The listing builds one solid part. Answer for the finished solid, in the listing's coordinates (mm). A direction names the side the tool comes from. Round coordinates to 2 decimals unless told otherwise and drop trailing zeros. Write each loop counter-clockwise with the first axis right and the second up, starting at its lowest first coordinate (ties: lowest second). Pieces come first, ordered by that corner, then holes.
Item 1: Find section B-B on x = 15.5. Give the vertices of the cut face in (y, z).
Item 2: A tool of negligible diameter and unlimited length cuts with its end or side. For faces 5 (the face through (15.023, -37.648, 1.014)), 6 (the face through (0, 1, -1)), from which of +Z, -Z, +X, -X, +Y, -Y can it reach the whole face along a straight path? Write none if from no direction.
Item 3: Find section C-C on z = -0.45. Give the vertices of the cut face in (x, y), then the cut area to 3 significant figures.
Item 4: Each of these flat-tipped pins is pushed along its axis until it touches: pin 1 (0.8 mm diameter, centred on x = -5, z = -0.5, fed in from -Y); pin 2 (1.3 mm diameter, centred on x = -16.5, y = 35.5, fed in from +Z). Where does it stop, or does it pass through?
Item 5: Find section D-D on y = 9. Give the vertices of the cut face in (x, z), then the cut area to 3 significant figures.
Item 6: Find section A-A on y = -35.5. Give the vertices of the cut face in (x, z), then the cut area to 3 significant figures.
Item 7: Find the intervals of material crossed by probe 1 along X at (y, z) = (-13.5, -0.45); probe 2 along Z at (x, y) = (18, -25); probe 3 along Y at (x, z) = (-12, -0.15), in increasing order.
Item 8: For a pull along Y with two mould halves and no side action, classify faces 1 (the face through (-18, 0, 0)), 2 (the face through (0, 40, 1)), 3 (the face through (0, -40, 1)), 4 (the face through (-15.66, 36.69, -0.49)) as +Y half, -Y half, draft (parallel to the pull), parting line (faces both ways), or undercut.
```python
from build123d import *

# Parameters (mm, degrees)
ESQUISSE1_W             = 40
ESQUISSE1_H             = 80
ESQUISSE1_W_2           = 35.6
ESQUISSE1_H_2           = 75.6
BOSS_EXTRU_1_DEPTH      = 2
ESQUISSE1_3_W           = 35.6
ESQUISSE1_3_H           = 75.6
BOSS_EXTRU_2_DEPTH      = 1
ESQUISSE2_R             = 1.2
ENL_V_MAT_EXTRU_1_DEPTH = 45.821869662
ESQUISSE2_3_R           = 2.2
ESQUISSE2_3_R_2         = 1.2
ENL_V_MAT_EXTRU_2_DEPTH = 2


with BuildPart() as part:
    # Esquisse1 → Boss.-Extru.1 (new body)
    # profile 1 of 2: a face of its own
    with BuildSketch(Plane.XY):
        Rectangle(ESQUISSE1_W, ESQUISSE1_H)
        Rectangle(ESQUISSE1_W_2, ESQUISSE1_H_2, mode=Mode.SUBTRACT)
    # profile 2 of 2: a face of its own
    with BuildSketch(Plane.XY):
        Rectangle(ESQUISSE1_W_2, ESQUISSE1_H_2)
    extrude(amount=BOSS_EXTRU_1_DEPTH)

    # Esquisse1_3 → Boss.-Extru.2 (add)
    with BuildSketch(Plane.XY):
        Rectangle(ESQUISSE1_3_W, ESQUISSE1_3_H)
    extrude(amount=-BOSS_EXTRU_2_DEPTH)

    # Esquisse2 → Enl_v. mat.-Extru.1 (cut, through all)
    with BuildSketch(Plane.XY.offset(2)):
        with Locations((-15.5, 35.5)):
            Circle(ESQUISSE2_R)
        with Locations((15.5, -35.5)):
            Circle(ESQUISSE2_R)
    extrude(amount=-ENL_V_MAT_EXTRU_1_DEPTH, mode=Mode.SUBTRACT)

    # Esquisse2_3 → Enl_v. mat.-Extru.2 (cut)
    # profile 1 of 2: a face of its own
    with BuildSketch(Plane.XY.offset(2)):
        with Locations((-15.5, 35.5)):
            Circle(ESQUISSE2_3_R)
        with Locations((-15.5, 35.5)):
            Circle(ESQUISSE2_3_R_2, mode=Mode.SUBTRACT)
    # profile 2 of 2: a face of its own
    with BuildSketch(Plane.XY.offset(2)):
        with Locations((15.5, -35.5)):
            Circle(ESQUISSE2_3_R)
        with Locations((15.5, -35.5)):
            Circle(ESQUISSE2_3_R_2, mode=Mode.SUBTRACT)
    extrude(amount=-ENL_V_MAT_EXTRU_2_DEPTH, mode=Mode.SUBTRACT)


solid = part.part
```
Check values:
1. outline: (-40, 0) - (-37.8, 0) - (-37.8, -1) - (-36.7, -1) - (-36.7, 0) - (-37.7, 0) - (-37.7, 2) - (-40, 2) - close; (-34.3, -1) - (37.8, -1) - (37.8, 0) - (40, 0) - (40, 2) - (-33.3, 2) - (-33.3, 0) - (-34.3, 0) - close
2. face 5: +Z
2. face 6: -Z, +X, -X, +Y, -Y
3. outline: (-17.8, -37.8) - (17.8, -37.8) - (17.8, 37.8) - (-17.8, 37.8) - close; hole circle Ø2.4 at (-15.5, 35.5); hole circle Ø2.4 at (15.5, -35.5)
3. area: 2,680 mm2
4. pin 1: stops at y = -37.8
4. pin 2: stops at z = 0
5. outline: (-20, 0) - (-17.8, 0) - (-17.8, -1) - (17.8, -1) - (17.8, 0) - (20, 0) - (20, 2) - (-20, 2) - close
5. area: 116 mm2
6. outline: (-20, 0) - (-17.8, 0) - (-17.8, -1) - (14.3, -1) - (14.3, 0) - (13.3, 0) - (13.3, 2) - (-20, 2) - close; (16.7, -1) - (17.8, -1) - (17.8, 0) - (20, 0) - (20, 2) - (17.7, 2) - (17.7, 0) - (16.7, 0) - close
6. area: 104 mm2
7. probe 1: x = -17.8 to 17.8
7. probe 2: z = 0 to 2
7. probe 3: y = -37.8 to 37.8
8. face 1: draft
8. face 2: +Y half
8. face 3: -Y half
8. face 4: undercut
